from build123d import *

# Parameters (mm, degrees)
SKETCH_1_R          = 25
EXTRUDE_1_DEPTH     = 4
SKETCH_2_R          = 4.25
EXTRUDE_2_DEPTH     = 72
SKETCH_3_R          = 2
CUT_EXTRUDE_1_DEPTH = 100


with BuildPart() as part:
    # 草图1 → 凸台-拉伸1 (new body)
    with BuildSketch(Plane.XY):
        Circle(SKETCH_1_R)
    extrude(amount=EXTRUDE_1_DEPTH)

    # 草图2 → 凸台-拉伸2 (add)
    with BuildSketch(Plane(origin=(0, 0, 0), x_dir=(-1, 0, 0), z_dir=(0, 0, -1))):
        with Locations((0.21687177, 0)):
            Circle(SKETCH_2_R)
    extrude(amount=EXTRUDE_2_DEPTH)

    # 草图3 → 切除-拉伸1 (cut)
    with BuildSketch(Plane(origin=(0, 0, 0), x_dir=(-1, 0, 0), z_dir=(0, 0, -1))):
        with Locations((0, 17.25)):
            Circle(SKETCH_3_R)
        with Locations((14.938938215, 8.625)):
            Circle(SKETCH_3_R)
        with Locations((14.938938215, -8.625)):
            Circle(SKETCH_3_R)
        with Locations((0, -17.25)):
            Circle(SKETCH_3_R)
        with Locations((-14.938938215, -8.625)):
            Circle(SKETCH_3_R)
        with Locations((-14.938938215, 8.625)):
            Circle(SKETCH_3_R)
    extrude(amount=-CUT_EXTRUDE_1_DEPTH, mode=Mode.SUBTRACT)


solid = part.part
Geometry: final body of the model. Coordinates: model frame, mm. Give positions to 0.01 mm unless a question says otherwise; leave off trailing zeros. Order: outer loops, then holes, each group sorted by start corner. A loop starts at its lowest first (then second) coordinate and runs counter-clockwise, first axis right, second up. Notation, with made-up numbers: (-30.75, -22.75) -> (23.25, -22.75) arc R15 cw to (23.25, 1.25) -> close; hole circle Ø7 at (-20.75, -7). An arc over 180 degrees is marked (long way). Answer as a JSON object with one key per item and string values.
Q1. Section B-B (x = 0). Output: boundary loops of the cut face in (y, z), plus the area to 3 significant figures.
Entries:
{"outline": "(-25, 0) -> (-19.25, 0) -> (-19.25, 4) -> (-25, 4) -> close; (-15.25, 0) -> (-4.24, 0) -> (-4.24, -72) -> (4.24, -72) -> (4.24, 0) -> (15.25, 0) -> (15.25, 4) -> (-15.25, 4) -> close; (19.25, 0) -> (25, 0) -> (25, 4) -> (19.25, 4) -> close", "area": "779 mm^2"}
Q2. First-contact query: pin 1 (3 mm diameter, centred on x = -5.5, z = -37.5, fed in from +Y); pin 2 (4.5 mm diameter, centred on x = 14.94, y = -8.62, fed in from -Z); pin 3 (12 mm diameter, centred on x = -1.5, z = -40, fed in from +Y). Flat tips, straight axial feed; report the tip coordinate or a pass-through.
Entries:
{"pin 1": "stops at y = 1.94", "pin 2": "stops at z = 0", "pin 3": "stops at y = 4.25"}
Q3. Section D-D (x = 6.5). Output: boundary loops of the cut face in (y, z), plus the area to 3 significant figures.
Entries:
{"outline": "(-24.14, 0) -> (24.14, 0) -> (24.14, 4) -> (-24.14, 4) -> close", "area": "193 mm^2"}
Q4. Section C-C (z = -61.5). Output: boundary loops of the cut face in (x, y), plus the area to 3 significant figures.
Entries:
{"outline": "circle Ø8.5 at (-0.22, 0)", "area": "56.7 mm^2"}
Q5. Material intervals for probe 1 along Y at (x, z) = (0, 1.8); probe 2 along Z at (x, y) = (-19.5, -11); probe 3 along X at (y, z) = (-2, -37.5), sorted ascending.
Entries:
{"probe 1": "y = -25 to -19.25, -15.25 to 15.25, 19.25 to 25", "probe 2": "z = 0 to 4", "probe 3": "x = -3.97 to 3.53"}
Q6. Draft query along Y for faces 1 (the cylindrical face through (-12.94, -8.54, 1.97)), 2 (the flat face through (0, -5, 0)), 3 (the cylindrical face through (0.336, 4.214, -35.496)). Return one class per face: released by +Y, released by -Y, zero draft, split by the parting line, or undercut.
Entries:
{"face 1": "undercut", "face 2": "zero draft", "face 3": "split by the parting line"}
Q7. Section A-A (y = 0). Output: boundary loops of the cut face in (x, z), plus the area to 3 significant figures.
Entries:
{"outline": "(-25, 0) -> (-4.47, 0) -> (-4.47, -72) -> (4.03, -72) -> (4.03, 0) -> (25, 0) -> (25, 4) -> (-25, 4) -> close", "area": "812 mm^2"}
